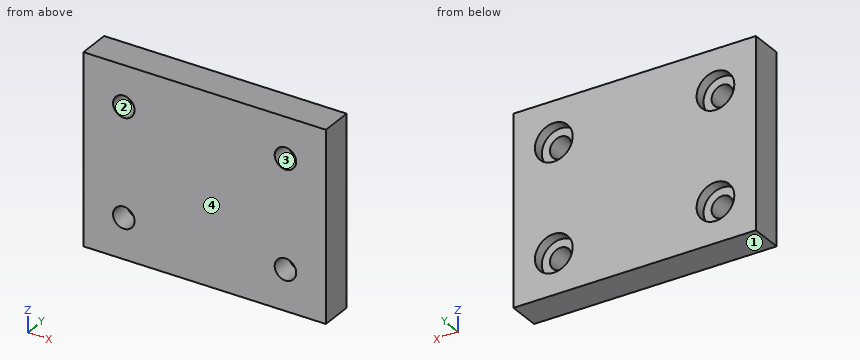
```python
from build123d import *

# Parameters (mm, degrees)
SKETCH_1_W          = 90
SKETCH_1_H          = 70
EXTRUDE_1_DEPTH     = 12
SKETCH_2_R          = 7
CUT_EXTRUDE_1_DEPTH = 4
SKETCH_3_R          = 4
CUT_EXTRUDE_2_DEPTH = 59.258046655


with BuildPart() as part:
    # 草图1 → 凸台-拉伸1 (new body)
    with BuildSketch(Plane(origin=(0, 0, 0), x_dir=(1, 0, 0), z_dir=(0, 1, 0))):
        Rectangle(SKETCH_1_W, SKETCH_1_H)
    extrude(amount=EXTRUDE_1_DEPTH)

    # 草图2 → 切除-拉伸1 (cut)
    with BuildSketch(Plane(origin=(0, 12, 0), x_dir=(1, 0, 0), z_dir=(0, 1, 0))):
        with Locations(Location((-30, 20, 0), (0, 0, 270))):
            Circle(SKETCH_2_R)
        with Locations(Location((30, 20, 0), (0, 0, 270))):
            Circle(SKETCH_2_R)
        with Locations(Location((-30, -20, 0), (0, 0, 270))):
            Circle(SKETCH_2_R)
        with Locations(Location((30, -20, 0), (0, 0, 270))):
            Circle(SKETCH_2_R)
    extrude(amount=-CUT_EXTRUDE_1_DEPTH, mode=Mode.SUBTRACT)

    # 草图3 → 切除-拉伸2 (cut, through all)
    with BuildSketch(Plane(origin=(0, 12, 0), x_dir=(1, 0, 0), z_dir=(0, 1, 0))):
        with Locations(Location((-30, 20, 0), (0, 0, 270))):
            Circle(SKETCH_3_R)
        with Locations(Location((30, 20, 0), (0, 0, 270))):
            Circle(SKETCH_3_R)
        with Locations(Location((-30, -20, 0), (0, 0, 270))):
            Circle(SKETCH_3_R)
        with Locations(Location((30, -20, 0), (0, 0, 270))):
            Circle(SKETCH_3_R)
    extrude(amount=-CUT_EXTRUDE_2_DEPTH, mode=Mode.SUBTRACT)


solid = part.part
```
The listing builds one solid part. Answer for the finished solid, in the listing's coordinates (mm). Face numbers are marked on the shaded views. Coordinates: 2 decimals unless noted, no trailing zeros. Write each loop counter-clockwise with the first axis right and the second up, starting at its lowest first coordinate (ties: lowest second). Pieces come first, ordered by that corner, then holes. Notation, with made-up numbers: M 85,-15 L 89,-15 A22 ccw 89,-7 Z; hole C -5,78 d7. An arc over 180 degrees is marked long. Use a Markdown table: item, result. Add a question column.
1. Section B-B (y = 3.75) is taken. Give the vertices of the cut face in (x, z).
2. For a pull along Z with two mould halves and no side action, classify the marked faces 1, 2, 3 and 4 as +Z half, -Z half, draft (parallel to the pull), parting line (faces both ways), or undercut.
3. Section C-C (z = -20) is taken. Give the vertices of the cut face in (x, y), plus the area to 3 significant figures.
4. Given P1, Ø13, axis at x = -30, z = -20, coming from the +Y side, flat-ended and moving along its own axis, determine where the tip first touches the part or whether it passes through.
5. Straight lines are drawn through the part: line 1 along X through (y, z) = (5, -20); line 2 along X through (y, z) = (10.55, -20); line 3 along Y through (x, z) = (30.5, 16). For each, find the intervals that lie inside material, in ascending order. Write a range as [from, to].
6. Section A-A (x = -30) is taken. Give the vertices of the cut face in (y, z), plus the area to 3 significant figures.
7. Section D-D (y = 10.5) is taken. Give the vertices of the cut face in (x, z).
Data:
| question | item | result |
|---|---|---|
| 1 | outline | M -45,-35 L 45,-35 L 45,35 L -45,35 Z; hole C -30,-20 d8; hole C -30,20 d8; hole C 30,-20 d8; hole C 30,20 d8 |
| 2 | face 1 | -Z half |
| 2 | face 2 | undercut |
| 2 | face 3 | undercut |
| 2 | face 4 | draft |
| 3 | outline | M -45,0 L -34,0 L -34,8 L -37,8 L -37,12 L -45,12 Z; M -26,0 L 26,0 L 26,8 L 23,8 L 23,12 L -23,12 L -23,8 L -26,8 Z; M 34,0 L 45,0 L 45,12 L 37,12 L 37,8 L 34,8 Z |
| 3 | area | 840 mm2 |
| 4 | P1 | stops at y = 8 |
| 5 | line 1 | x = [-45, -34], [-26, 26], [34, 45] |
| 5 | line 2 | x = [-45, -37], [-23, 23], [37, 45] |
| 5 | line 3 | y = [0, 8] |
| 6 | outline | M 0,-35 L 12,-35 L 12,-27 L 8,-27 L 8,-24 L 0,-24 Z; M 0,-16 L 8,-16 L 8,-13 L 12,-13 L 12,13 L 8,13 L 8,16 L 0,16 Z; M 0,24 L 8,24 L 8,27 L 12,27 L 12,35 L 0,35 Z |
| 6 | area | 600 mm2 |
| 7 | outline | M -45,-35 L 45,-35 L 45,35 L -45,35 Z; hole C -30,-20 d14; hole C -30,20 d14; hole C 30,-20 d14; hole C 30,20 d14 |
